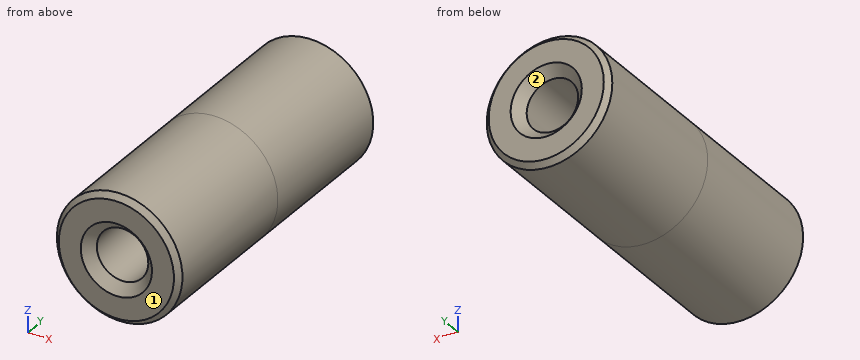
Autodesk Inventor part; units mm, degrees
ref_plane "YZ Plane" through (0, 0, 0) normal (1, 0, 0) x (0, 1, 0)
ref_plane "XZ Plane" through (0, 0, 0) normal (0, 1, 0) x (-1, 0, 0)
ref_plane "XY Plane" through (0, 0, 0) normal (0, 0, 1) x (1, 0, 0)
sketch "スケッチ1" plane through (0, 0, 0) normal (0, 1, 0) x (-1, 0, 0)
  circle A0 centre (0, 0) radius 3
  dimension "d0" = 6
extrude "押し出し1" add sketch "スケッチ1" along normal mid plane 15
sketch "スケッチ2" plane through (0, 7.5, 0) normal (0, 1, 0) x (1, 0, 0)
  point P0 (0, 0)
  point P1 (0, 0)
hole "穴1" at (0, 7.5, 0) direction (0, -1, 0) diameter 2.459 depth 10 countersink diameter 3.4 countersink angle 90
sketch "スケッチ3" plane through (0, -7.5, 0) normal (0, -1, 0) x (1, 0, 0)
  point P0 (0, 0)
  point P1 (0, 0)
hole "穴2" at (0, -7.5, 0) direction (0, 1, 0) diameter 2.459 depth 10 countersink diameter 3.4 countersink angle 90
chamfer "面取り1" distance 0.25 angle 45 2 edges at (3, -7.5, 0) (3, 7.5, 0)
properties part number "Spacer_M3D6L60" material "アルミニウム 6061"
For this review, take the finished solid that the model builds, in its own axes (mm). Face numbers are marked on the shaded views. Coordinates: 2 decimals unless noted, no trailing zeros. Loops run counter-clockwise (first coordinate to the right, second up) from the corner with the lowest first, then second, coordinate; pieces in that order, holes last.
1. Add section B-B, the plane y = 6.5. Give the boundary of the cut face in (x, z), then the cut area to 3 significant figures.
2. Add section A-A, the plane z = 0. Give the boundary of the cut face in (x, y), then the cut area to 3 significant figures.
3. Mouldability with a two-part tool opening along Z and no side actions: class the marked faces 1 and 2 as +Z half, -Z half, draft (parallel to the pull), parting line (faces both ways), or undercut.
4. For line 1 (Z direction, x = 0, y = -5.5); line 2 (Z direction, x = -0.95, y = -5.5); line 3 (X direction, y = 1, z = -1.05), list the stretches that pass through material, from the lowest coordinate up.
5. Insertion check: P1, Ø3, axis at x = 0.5, y = -6, coming from the -Z side; P2, Ø1.5, axis at y = -1.5, z = 1.5, coming from the +X side. Each pin has a flat end and moves straight along its axis. Give the tip position at first contact, or say it passes through.
Result:
1. outline: circle Ø6 at (0, 0); hole circle Ø2.46 at (0, 0)
1. area: 23.5 mm2
2. outline: (-3, -7.25) - (-2.75, -7.5) - (-1.7, -7.5) - (-1.23, -7.03) - (-1.23, 7.03) - (-1.7, 7.5) - (-2.75, 7.5) - (-3, 7.25) - close; (1.23, -7.03) - (1.7, -7.5) - (2.75, -7.5) - (3, -7.25) - (3, 7.25) - (2.75, 7.5) - (1.7, 7.5) - (1.23, 7.03) - close
2. area: 52.5 mm2
3. face 1: draft
3. face 2: undercut
4. line 1: z = -3 to -1.23, 1.23 to 3
4. line 2: z = -2.85 to -0.78, 0.78 to 2.85
4. line 3: x = -2.81 to -0.64, 0.64 to 2.81
5. P1: stops at z = -3
5. P2: stops at x = 2.9
